Verification items for the finished model (mm, model axes). Give positions to 0.01 mm unless a question says otherwise; leave off trailing zeros. Write each loop counter-clockwise with the first axis right and the second up, starting at its lowest first coordinate (ties: lowest second). Pieces come first, ordered by that corner, then holes. Notation, with made-up numbers: M 14.25,86 L 23.25,86 A18 ccw 23.25,112 Z; hole C 56.5,52.25 d6. An arc over 180 degrees is marked long. Write item = value, one per line.
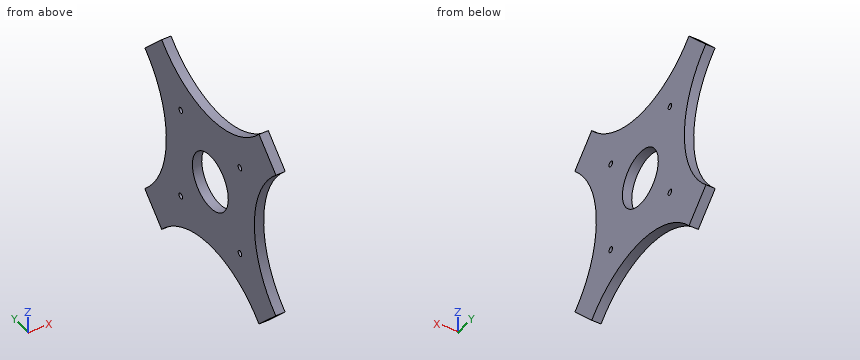
from build123d import *

# Parameters (mm, degrees)
SKETCH_1_R      = 15
SKETCH_1_R_2    = 1.5
EXTRUDE_1_DEPTH = 5


with BuildPart() as part:
    # 草图1 → 凸台-拉伸1 (new body)
    with BuildSketch(Plane(origin=(0, 0, 0), x_dir=(0, 0, -1), z_dir=(1, 0, 0))):
        with BuildLine():
            Line((-54.891168705, 40.66351007), (-40.699692853, 54.756132721))
            ThreePointArc((-40.699692853, 54.756132721), (0.011760124, 36.837223596), (40.66351007, 54.891168705))
            Line((40.66351007, 54.891168705), (54.756132721, 40.699692853))
            ThreePointArc((54.756132721, 40.699692853), (36.837223596, -0.011760124), (54.891168705, -40.66351007))
            Line((54.891168705, -40.66351007), (40.699692853, -54.756132721))
            ThreePointArc((40.699692853, -54.756132721), (-0.011760124, -36.837223596), (-40.66351007, -54.891168705))
            Line((-40.66351007, -54.891168705), (-54.756132721, -40.699692853))
            ThreePointArc((-54.756132721, -40.699692853), (-36.837223596, 0.011760124), (-54.891168705, 40.66351007))
        make_face()
        Circle(SKETCH_1_R, mode=Mode.SUBTRACT)
        with Locations((24.748737342, 24.748737342)):
            Circle(SKETCH_1_R_2, mode=Mode.SUBTRACT)
        with Locations((24.748737342, -24.748737342)):
            Circle(SKETCH_1_R_2, mode=Mode.SUBTRACT)
        with Locations((-24.748737342, -24.748737342)):
            Circle(SKETCH_1_R_2, mode=Mode.SUBTRACT)
        with Locations((-24.748737342, 24.748737342)):
            Circle(SKETCH_1_R_2, mode=Mode.SUBTRACT)
    extrude(amount=EXTRUDE_1_DEPTH)


solid = part.part
1) Depth check by flat-ended pin: P1, Ø2.5, axis at y = 24.75, z = -24.75, coming from the -X side; P2, Ø2, axis at x = 2, z = -5, coming from the +Y side; P3, Ø2, axis at x = 4, y = -22, coming from the +Z side; P4, Ø1, axis at y = 17.5, z = -29.5, coming from the -X side. Enter the tip coordinate at first touch or a pass-through.
From the geometry:
P1 = through
P2 = 37.17
P3 = 41.84
P4 = 0
2) Cross-section at A-A on y = 3. Record the boundary of the cut face in (x, z).
From the geometry:
outline = M 0,-36.91 L 5,-36.91 L 5,-14.7 L 0,-14.7 Z; M 0,14.7 L 5,14.7 L 5,36.92 L 0,36.92 Z
3) Cross-section at C-C on x = 1. Record the boundary of the cut face in (y, z), plus the area to 3 significant figures.
From the geometry:
outline = M -54.89,40.66 A55 cw -54.76,-40.7 L -40.66,-54.89 A55 cw 40.7,-54.76 L 54.89,-40.66 A55 cw 54.76,40.7 L 40.66,54.89 A55 cw -40.7,54.76 Z; hole C -24.75,-24.75 d3; hole C -24.75,24.75 d3; hole C 0,0 d30; hole C 24.75,-24.75 d3; hole C 24.75,24.75 d3
area = 6,840 mm^2
4) Material ranges on probe 1 along Y at (x, z) = (1.4, 0); probe 2 along Z at (x, y) = (3.55, -42); probe 3 along Z at (x, y) = (3.35, -12), recorded low to high. Write a range as from..to.
From the geometry:
probe_1 = -36.84..-15, 15..36.84
probe_2 = -53.55..-23.34, 23.19..53.46
probe_3 = -38.18..-9, 9..38.14
5) Cross-section at D-D on z = 30. Record the boundary of the cut face in (x, y), plus the area to 3 significant figures.
From the geometry:
outline = M 0,-45.79 L 5,-45.79 L 5,45.69 L 0,45.69 Z
area = 457 mm^2
6) Cross-section at B-B on z = 0. Record the boundary of the cut face in (x, y).
From the geometry:
outline = M 0,-36.84 L 5,-36.84 L 5,-15 L 0,-15 Z; M 0,15 L 5,15 L 5,36.84 L 0,36.84 Z
